Build history of the part. All positions in model axes, mm. A direction names the side the tool comes from. Give positions to 0.01 mm unless a question says otherwise; leave off trailing zeros. Order: outer loops, then holes, each group sorted by start corner. A loop starts at its lowest first (then second) coordinate and runs counter-clockwise, first axis right, second up. Notation, with made-up numbers: (49.25, 33.5) - (101.25, 33.5) arc R35 cw to (101.25, 72.5) - close; hole circle Ø5 at (-30, 22). An arc over 180 degrees is marked (long way). Write each question's results on one line, items separated by ' | '. Start each with the question number.
1) Cut at D-D on y = 2.1. List the corners of the cut face in (x, z).
2) Drill centre lines: line 1 along Z through (x, y) = (-1.65, -1); line 2 along Y through (x, z) = (0.85, 1.15); line 3 along X through (y, z) = (-0.1, 0.4). Where is each one in solid material? Low to high. Write a range as from..to.
3) Tool access for faces 1 (the face through (1.25, 1.25, 0.1)), 2 (the face through (1.25, -1.25, 2.4)): list every direction of +Z, -Z, +X, -X, +Y, -Y with a clear straight run to the whole face (end or side of a thin tool).
4) Two-plate mould, pull along X, no slides. Class faces 3 (the face through (-3, 0, 1)), 4 (the face through (-1.5, 0.07, 1.23)): +X half, -X half, draft (parallel to the pull), parting line (faces both ways), or undercut.
5) Drop flat-ended pins along their axis: pin 1 Ø3 at (x, y) = (1.5, 1) entering from -Z; pin 2 Ø1.5 at (x, z) = (-2.5, 1.5) entering from -Y. Give the stop position or say it passes through.
6) Cut at C-C on z = 1.1. List the corners of the cut face in (x, y), plus the area to 3 significant figures.
7) Cut at A-A on x = 0. List the corners of the cut face in (y, z), plus the area to 3 significant figures.
from build123d import *

# Parameters (mm, degrees)
CROQUIS1_R                = 1.6
CROQUIS1_R_2              = 1.5
SALIENTE_EXTRUIR1_DEPTH   = 2.5
CROQUIS1_R_3              = 3
CROQUIS1_R_4              = 2.9
SALIENTE_EXTRUIR1_2_DEPTH = 2.5
CROQUIS2_R                = 2.9
CROQUIS2_R_2              = 1.6
SALIENTE_EXTRUIR4_DEPTH   = 2.4
CROQUIS3_R                = 2.9
CROQUIS3_R_2              = 1.6
CORTAR_EXTRUIR1_DEPTH     = 0.1


with BuildPart() as part:
    # Croquis1 → Saliente-Extruir1 (new body)
    with BuildSketch(Plane.XY):
        Circle(CROQUIS1_R)
        Circle(CROQUIS1_R_2, mode=Mode.SUBTRACT)
    extrude(amount=SALIENTE_EXTRUIR1_DEPTH)



with BuildPart() as body_2:
    # Croquis1 → Saliente-Extruir1 2 (new body)
    with BuildSketch(Plane.XY):
        Circle(CROQUIS1_R_3)
        Circle(CROQUIS1_R_4, mode=Mode.SUBTRACT)
    extrude(amount=SALIENTE_EXTRUIR1_2_DEPTH)


with BuildPart() as part_1:
    add(part.part)

    add(body_2.part)  # Saliente-Extruir4 merges body 2
    # Croquis2 → Saliente-Extruir4 (add)
    with BuildSketch(Plane.XY):
        Circle(CROQUIS2_R)
        Circle(CROQUIS2_R_2, mode=Mode.SUBTRACT)
    extrude(amount=SALIENTE_EXTRUIR4_DEPTH)

    # Croquis3 → Cortar-Extruir1 (cut)
    with BuildSketch(Plane(origin=(0, 0, 0), x_dir=(-1, 0, 0), z_dir=(0, 0, -1))):
        with Locations(Location((0, 0, 0), (0, 0, 180))):
            Circle(CROQUIS3_R)
        with Locations(Location((0, 0, 0), (0, 0, 180))):
            Circle(CROQUIS3_R_2, mode=Mode.SUBTRACT)
    extrude(amount=-CORTAR_EXTRUIR1_DEPTH, mode=Mode.SUBTRACT)


solid = part_1.part
Results:
1) outline: (-2.14, 0) - (-2, 0) - (-2, 0.1) - (2, 0.1) - (2, 0) - (2.14, 0) - (2.14, 2.5) - (2, 2.5) - (2, 2.4) - (-2, 2.4) - (-2, 2.5) - (-2.14, 2.5) - close
2) line 1: 0.1..2.4 | line 2: -2.88..-1.24, 1.24..2.88 | line 3: -3..-1.5, 1.5..3
3) face 1: -Z | face 2: +Z
4) face 3: parting line | face 4: undercut
5) pin 1: z = 0 | pin 2: y = -2.44
6) outline: circle Ø6 at (0, 0); hole circle Ø3 at (0, 0) | area: 21.2 mm^2
7) outline: (-3, 0) - (-2.9, 0) - (-2.9, 0.1) - (-1.6, 0.1) - (-1.6, 0) - (-1.5, 0) - (-1.5, 2.5) - (-1.6, 2.5) - (-1.6, 2.4) - (-2.9, 2.4) - (-2.9, 2.5) - (-3, 2.5) - close; (1.5, 0) - (1.6, 0) - (1.6, 0.1) - (2.9, 0.1) - (2.9, 0) - (3, 0) - (3, 2.5) - (2.9, 2.5) - (2.9, 2.4) - (1.6, 2.4) - (1.6, 2.5) - (1.5, 2.5) - close | area: 6.98 mm^2
